Could you check a few things on this drawing? It's one solid part, dimensions in mm from its lowest x, y, z. Give positions to 0.01 mm unless a question says otherwise; leave off trailing zeros. Order: outer loops, then holes, each group sorted by start corner. A loop starts at its lowest first (then second) coordinate and runs counter-clockwise, first axis right, second up.
Item 1: I'm going to push flat-ended pins straight in: pin 1 Ø3 at (x, y) = (6.35, 57.15) entering from +Z; pin 2 Ø0.8 at (x, z) = (17.5, 1) entering from -Y; pin 3 Ø0.8 at (y, z) = (17.5, 1) entering from -X. Where does each tip first touch, or does it pass through?
Item 2: I want a section at A-A, the plane y = 31.75. Write out the boundary of the cut face in (x, z).
Item 3: I want a section at D-D, the plane y = 58. Write out the boundary of the cut face in (x, z).
Item 4: I want a section at B-B, the plane z = 1.1. Count the separate pieces of the cut face and the enclosed holes in it, then the cut area to 3 significant figures.
Item 5: If I drill on line 1 along Y through (x, z) = (57.15, 0.8); line 2 along Y through (x, z) = (6.35, 0.95); line 3 along X through (y, z) = (44, 1.1), over which ranges is the centre line in solid material (lowest first)?
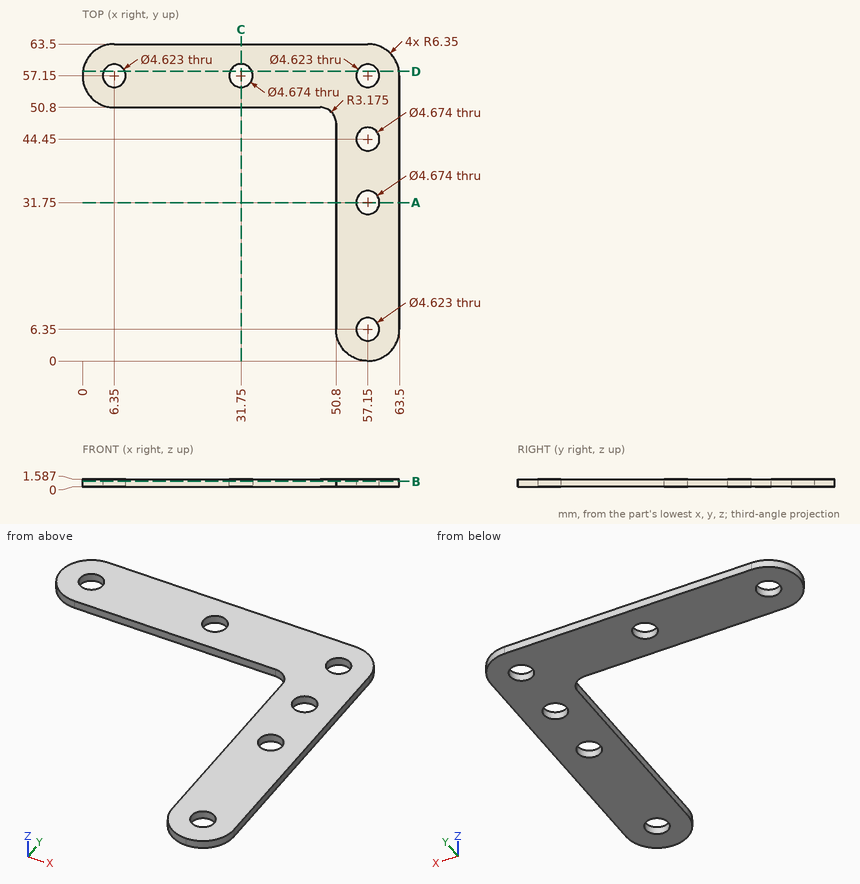
Results list:
1. pin 1: passes through
1. pin 2: stops at y = 50.8
1. pin 3: stops at x = 50.8
2. outline: (50.8, 0) - (54.81, 0) - (54.81, 1.59) - (50.8, 1.59) - close; (59.49, 0) - (63.5, 0) - (63.5, 1.59) - (59.49, 1.59) - close
3. outline: (0.06, 0) - (4.2, 0) - (4.2, 1.59) - (0.06, 1.59) - close; (8.5, 0) - (29.57, 0) - (29.57, 1.59) - (8.5, 1.59) - close; (33.93, 0) - (55, 0) - (55, 1.59) - (33.93, 1.59) - close; (59.3, 0) - (63.44, 0) - (63.44, 1.59) - (59.3, 1.59) - close
4. separate pieces: 1
4. enclosed holes: 6
4. area: 1,310 mm2
5. line 1: y = 0 to 4.04, 8.66 to 29.41, 34.09 to 42.11, 46.79 to 54.84, 59.46 to 63.5
5. line 2: y = 50.8 to 54.84, 59.46 to 63.5
5. line 3: x = 50.8 to 54.86, 59.44 to 63.5
